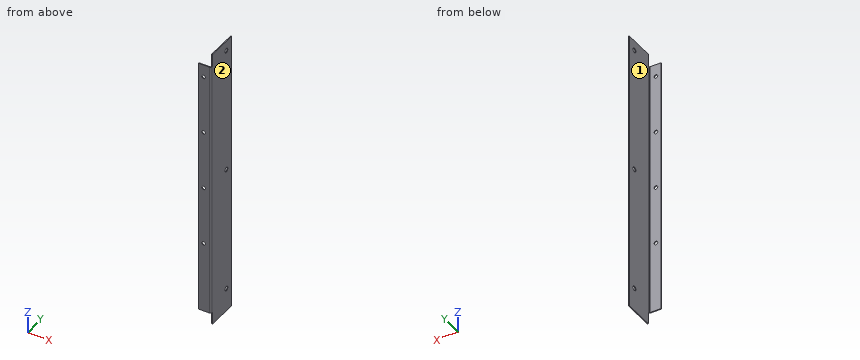
from build123d import *

# Parameters (mm, degrees)
EXTRUDE_1_DEPTH     = 340
SKETCH_2_R          = 2.8
CUT_EXTRUDE_1_DEPTH = 340
SKETCH_3_R          = 2.15
CUT_EXTRUDE_2_DEPTH = 340
SKETCH_4_W          = 37.623292197
SKETCH_4_H          = 20.655925128
SKETCH_4_W_2        = 42.547460075
SKETCH_4_H_2        = 15
SKETCH_4_W_3        = 34.50961452
CUT_EXTRUDE_3_DEPTH = 3


with BuildPart() as part:
    # Эскиз1 → Вытянуть1 (new body)
    with BuildSketch(Plane.XY):
        with BuildLine():
            Line((-2, 0), (-15, 0))
            Line((-15, 0), (-15, 1))
            Line((-15, 1), (-2, 1))
            ThreePointArc((-2, 1), (-1.292893219, 1.292893219), (-1, 2))
            Line((-1, 2), (-1, 40))
            Line((-1, 40), (0, 40))
            Line((0, 40), (0, 2))
            ThreePointArc((0, 2), (-0.585786438, 0.585786438), (-2, 0))
        make_face()
    extrude(amount=-EXTRUDE_1_DEPTH)

    # Эскиз2 → Вырез-Вытянуть1 (cut)
    with BuildSketch(Plane(origin=(0, 0, 0), x_dir=(0, 0, -1), z_dir=(1, 0, 0))):
        with Locations((12, 30)):
            Circle(SKETCH_2_R)
        with Locations((162, 30)):
            Circle(SKETCH_2_R)
        with Locations((312, 30)):
            Circle(SKETCH_2_R)
    extrude(amount=-CUT_EXTRUDE_1_DEPTH, mode=Mode.SUBTRACT)

    # Эскиз3 → Вырез-Вытянуть2 (cut)
    with BuildSketch(Plane.XZ):
        with Locations((-9, -240)):
            Circle(SKETCH_3_R)
        with Locations((-9, -170)):
            Circle(SKETCH_3_R)
        with Locations((-9, -100)):
            Circle(SKETCH_3_R)
        with Locations((-9, -30)):
            Circle(SKETCH_3_R)
    extrude(amount=-CUT_EXTRUDE_2_DEPTH, mode=Mode.SUBTRACT)

    # Эскиз4 → Вырез-Вытянуть3 (cut)
    with BuildSketch(Plane.XZ):
        with Locations((6.462024168, 335.327962564)):
            Rectangle(SKETCH_4_W, SKETCH_4_H)
        with Locations((3.999940229, -7.5)):
            Rectangle(SKETCH_4_W_2, SKETCH_4_H_2)
        with Locations((2.25480726, -332.5)):
            Rectangle(SKETCH_4_W_3, SKETCH_4_H_2)
    extrude(amount=-CUT_EXTRUDE_3_DEPTH, mode=Mode.SUBTRACT)


solid = part.part
Design review of the part built by this model. Coordinates are the model's own, in mm. Face numbers are marked on the shaded views. A direction names the side the tool comes from. Give positions to 0.01 mm unless a question says otherwise; leave off trailing zeros. Loops run counter-clockwise (first coordinate to the right, second up) from the corner with the lowest first, then second, coordinate; pieces in that order, holes last. Notation, with made-up numbers: (68, 17.5) - (89, 17.5) arc R8 cw to (89, 29.5) - close; hole circle Ø2 at (75, -18). An arc over 180 degrees is marked (long way). Write item = value, one per line.
1) Take a section at B-B on z = -12. State the section outline as (x, y) points.
Result sheet:
outline = (-1, 3) - (0, 3) - (0, 27.2) - (-1, 27.2) - close; (-1, 32.8) - (0, 32.8) - (0, 40) - (-1, 40) - close
2) Clearance check with flat-ended pins moving along their axes: pin 1 Ø4 at (x, z) = (-9, -170) entering from -Y; pin 2 Ø5 at (x, z) = (-4, -86.5) entering from +Y; pin 3 Ø6.5 at (x, z) = (-8, -99.5) entering from +Y; pin 4 Ø0.8 at (x, z) = (-0.5, -330.5) entering from -Y. State where each tip first meets the part, or that it passes through.
Result sheet:
pin_1 = through
pin_2 = 1.13
pin_3 = 1
pin_4 = 3
3) Tool access review of the marked faces 1 and 2: name each direction out of +Z, -Z, +X, -X, +Y, -Y from which nothing blocks a thin tool from reaching the whole face with its end or side.
Result sheet:
face_1 = +Z, -Z, -X, +Y
face_2 = +Z, -Z, +X, +Y, -Y
4) Take a section at C-C on y = 7.5. State the section outline as (x, z) points.
Result sheet:
outline = (-1, -340) - (0, -340) - (0, 0) - (-1, 0) - close
5) To check wall thickness, follow line 1 (Z direction, x = -9, y = 0.6); line 2 (X direction, y = 34, z = -130); line 3 (Y direction, x = -3.25, z = -53.5). State the ranges of each line that lie inside material, in increasing order.
Result sheet:
line_1 = -325 to -242.15, -237.85 to -172.15, -167.85 to -102.15, -97.85 to -32.15, -27.85 to -15
line_2 = -1 to 0
line_3 = 0 to 1
6) Take a section at A-A on z = -162. State the section outline as (x, y) points, and give its area (3 significant figures).
Result sheet:
outline = (-15, 0) - (-2, 0) arc R2 ccw to (0, 2) - (0, 27.2) - (-1, 27.2) - (-1, 2) arc R1 cw to (-2, 1) - (-15, 1) - close; (-1, 32.8) - (0, 32.8) - (0, 40) - (-1, 40) - close
area = 47.8 mm2
